```python
from build123d import *

# Parameters (mm, degrees)
ESQUISSE1_R        = 30
ESQUISSE1_R_2      = 2.25
ESQUISSE1_R_3      = 4
BOSS_EXTRU_1_DEPTH = 5
ESQUISSE2_R        = 2.8
BOSS_EXTRU_2_DEPTH = 15


with BuildPart() as part:
    # Esquisse1 → Boss.-Extru.1 (new body)
    with BuildSketch(Plane.XY):
        Circle(ESQUISSE1_R)
        with Locations((18, 18)):
            Circle(ESQUISSE1_R_2, mode=Mode.SUBTRACT)
        with Locations((-18, 18)):
            Circle(ESQUISSE1_R_2, mode=Mode.SUBTRACT)
        with Locations((-18, -18)):
            Circle(ESQUISSE1_R_2, mode=Mode.SUBTRACT)
        with Locations((18, -18)):
            Circle(ESQUISSE1_R_2, mode=Mode.SUBTRACT)
        with Locations((18, 0)):
            Circle(ESQUISSE1_R_3, mode=Mode.SUBTRACT)
        with Locations((-18, 0)):
            Circle(ESQUISSE1_R_3, mode=Mode.SUBTRACT)
    extrude(amount=BOSS_EXTRU_1_DEPTH)

    # Esquisse2 → Boss.-Extru.2 (add)
    with BuildSketch(Plane(origin=(0, 0, 0), x_dir=(-1, 0, 0), z_dir=(0, 0, -1))):
        with BuildLine():
            Line((7.5, 12.5), (7.5, -12.5))
            ThreePointArc((7.5, -12.5), (0, -20), (-7.5, -12.5))
            Line((-7.5, -12.5), (-7.5, 12.5))
            ThreePointArc((-7.5, 12.5), (0, 20), (7.5, 12.5))
        make_face()
        with Locations((0, 12.5)):
            Circle(ESQUISSE2_R, mode=Mode.SUBTRACT)
        with Locations((0, -12.5)):
            Circle(ESQUISSE2_R, mode=Mode.SUBTRACT)
    extrude(amount=BOSS_EXTRU_2_DEPTH)


solid = part.part
```
CAD build for the part. Positions are in the model's coordinates, mm. A direction names the side the tool comes from. Give positions to 0.01 mm unless a question says otherwise; leave off trailing zeros. Order: outer loops, then holes, each group sorted by start corner. A loop starts at its lowest first (then second) coordinate and runs counter-clockwise, first axis right, second up. Notation, with made-up numbers: M 89,37.5 L 131,37.5 A17 cw 131,55.5 Z; hole C 43,3.5 d8. An arc over 180 degrees is marked long. Put each result on its own line as item: value. Start each with the question number.
(1) Flat gauge pins, fed straight in: pin 1 Ø8 at (x, z) = (-2.5, -6.5) entering from -Y; pin 2 Ø1.7 at (x, y) = (-1, -14) entering from -Z; pin 3 Ø4 at (y, z) = (-19, 0.5) entering from -X. Where does each tip first touch, or does it go through?
(2) Saw through at A-A, the plane x = -18. Write the cut outline in (y, z).
(3) Mould opens along X. For faces 5 (the cylindrical face through (-29.97, 1.32, 2.46)), 6 (the flat face through (0, 0, -15)), 7 (the flat face through (0, -12, 0)) say: +X half, -X half, draft (parallel to the pull), parting line (faces both ways), or undercut.
(4) Saw through at C-C, the plane z = -13.5. Write the cut outline in (x, y).
(5) Saw through at D-D, the plane x = 0. Write the cut outline in (y, z), then the cut area to 3 significant figures.
(6) Saw through at B-B, the plane z = 2.5. Write the cut outline in (x, y).
(7) Drill centre lines: line 1 along Y through (x, z) = (-1.5, -1.5); line 2 along Y through (x, z) = (-18, 2.1); line 3 along Z through (x, y) = (14, 22). Where is each one in solid material? Low to high.
(8) Which spindle directions (+Z, -Z, +X, -X, +Y, -Y) get a long thin tool onto all of the face, cutting with end or side? Do faces 1 (the cylindrical face through (0, 20, -7)), 2 (the flat face through (0, 13, 0)), 3 (the flat face through (7.5, 0, -7)), 4 (the flat face through (-7.5, 0, -7)). Say none if no direction does.
Check result:
1. pin 1: stops at y = -20
1. pin 2: stops at z = 0
1. pin 3: stops at x = -24.72
2. outline: M -24,0 L -20.25,0 L -20.25,5 L -24,5 Z; M -15.75,0 L -4,0 L -4,5 L -15.75,5 Z; M 4,0 L 15.75,0 L 15.75,5 L 4,5 Z; M 20.25,0 L 24,0 L 24,5 L 20.25,5 Z
3. face 5: parting line
3. face 6: draft
3. face 7: undercut
4. outline: M -7.5,-12.5 A7.5 ccw 7.5,-12.5 L 7.5,12.5 A7.5 ccw -7.5,12.5 Z; hole C 0,-12.5 d5.6; hole C 0,12.5 d5.6
5. outline: M -30,0 L -20,0 L -20,-15 L -15.3,-15 L -15.3,0 L -9.7,0 L -9.7,-15 L 9.7,-15 L 9.7,0 L 15.3,0 L 15.3,-15 L 20,-15 L 20,0 L 30,0 L 30,5 L -30,5 Z
5. area: 732 mm2
6. outline: C 0,0 d60; hole C -18,0 d8; hole C -18,-18 d4.5; hole C -18,18 d4.5; hole C 18,0 d8; hole C 18,-18 d4.5; hole C 18,18 d4.5
7. line 1: y = -19.85 to -14.86, -10.14 to 10.14, 14.86 to 19.85
7. line 2: y = -24 to -20.25, -15.75 to -4, 4 to 15.75, 20.25 to 24
7. line 3: z = 0 to 5
8. face 1: -Z, +Y
8. face 2: -Z
8. face 3: -Z, +X, +Y, -Y
8. face 4: -Z, -X, +Y, -Y
